The model under review builds one solid part; all positions refer to its coordinate system, in mm. A direction names the side the tool comes from. Coordinates: 2 decimals unless noted, no trailing zeros. Order: outer loops, then holes, each group sorted by start corner. A loop starts at its lowest first (then second) coordinate and runs counter-clockwise, first axis right, second up. Notation, with made-up numbers: M 26.25,9.5 L 84.25,9.5 A7 ccw 84.25,17.5 Z; hole C 77,30 d9. An arc over 180 degrees is marked long. Write each question's results on one line, items separated by ' | '.
from build123d import *

# Parameters (mm, degrees)
SKETCH1_W           = 120
SKETCH1_H           = 245
BOSS_EXTRUDE1_DEPTH = 42
CHAMFER1_SIZE       = 30
FILLET3_R           = 25
FILLET1_R           = 5
SHELL1_T            = -2


with BuildPart() as part:
    # Sketch1 → Boss-Extrude1 (new body)
    with BuildSketch(Plane.XY):
        with Locations((0, 72.5)):
            Rectangle(SKETCH1_W, SKETCH1_H)
    extrude(amount=BOSS_EXTRUDE1_DEPTH)

    # Chamfer1
    chamfer1_edges = [part.edges().sort_by_distance(p)[0] for p in [
        (60, -50, 21),
        (-60, -50, 21),
    ]]
    chamfer(chamfer1_edges, length=CHAMFER1_SIZE)

    # Fillet3
    fillet3_edges = [part.edges().sort_by_distance(p)[0] for p in [
        (30, -50, 21),
        (-30, -50, 21),
        (-60, -20, 21),
        (60, -20, 21),
    ]]
    fillet(fillet3_edges, radius=FILLET3_R)

    # Fillet1
    fillet1_edges = [part.edges().sort_by_distance(p)[0] for p in [
        (-45, -35, 0),
        (0, -50, 0),
        (60, 92.67766953, 0),
        (45, -35, 0),
        (58.096988313, -19.21174675, 0),
        (29.21174675, -48.096988313, 0),
        (-29.21174675, -48.096988313, 0),
        (-58.096988313, -19.21174675, 0),
        (0, 195, 0),
        (-60, 92.67766953, 0),
    ]]
    fillet(fillet1_edges, radius=FILLET1_R)

    # Shell1
    shell1_openings = [part.faces().sort_by_distance(p)[0] for p in [
        (0, 76.260599265, 42),
    ]]
    offset(amount=SHELL1_T, openings=shell1_openings)


solid = part.part
1) Take a section at B-B on x = 14. State the section outline as (y, z) points.
Solutions:
outline: M -50,5 A5 ccw -45,0 L 190,0 A5 ccw 195,5 L 195,42 L 193,42 L 193,5 A3 cw 190,2 L -45,2 A3 cw -48,5 L -48,42 L -50,42 Z
2) To check wall thickness, follow line 1 along Y through (x, z) = (-0.5, 6); line 2 along X through (y, z) = (132, 34); line 3 along Z through (x, y) = (18, -1.5). State the ranges of each line that lie inside material, in increasing order.
Solutions:
line 1: -50 to -48, 193 to 195 | line 2: -60 to -58, 58 to 60 | line 3: 0 to 2
3) Take a section at C-C on y = 23. State the section outline as (x, z) points, plus the area to 3 significant figures.
Solutions:
outline: M -60,5 A5 ccw -55,0 L 55,0 A5 ccw 60,5 L 60,42 L 58,42 L 58,5 A3 cw 55,2 L -55,2 A3 cw -58,5 L -58,42 L -60,42 Z | area: 393 mm2
4) For faces 5 (the cylindrical face through (58, 94, 1)), 6 (the flat face through (58, 90, 23)), list the 3-axis set-ups (+Z, -Z, +X, -X, +Y, -Y) from which the entire face can be reached by the end or side of a thin tool; tool diameter is ignored.
Solutions:
face 5: -Z, +X, +Y, -Y | face 6: +Z
5) For pin 1 (4 mm diameter, centred on x = 33.5, z = 22.5, fed in from -Y); pin 2 (5 mm diameter, centred on x = -17, y = 15, fed in from +Z), all flat-tipped, find the tip position at first contact; note any pin that passes through.
Solutions:
pin 1: y = -47.01 | pin 2: z = 2
6) Take a section at A-A on z = 26. State the section outline as (x, y) points.
Solutions:
outline: M -60,-9.64 A25 ccw -52.68,-27.32 L -37.32,-42.68 A25 ccw -19.64,-50 L 19.64,-50 A25 ccw 37.32,-42.68 L 52.68,-27.32 A25 ccw 60,-9.64 L 60,195 L -60,195 Z; hole M -58,-9.64 A23 ccw -51.26,-25.91 L -35.91,-41.26 A23 ccw -19.64,-48 L 19.64,-48 A23 ccw 35.91,-41.26 L 51.26,-25.91 A23 ccw 58,-9.64 L 58,193 L -58,193 Z
7) The part is to be moulded in two halves that separate along Y. For faces 1 (the flat face through (-1, 74, 0)), 2 (the cylindrical face through (1, 193, 1)), 3 (the cylindrical face through (-28.56, -46.2, 23.76)), 4 (the flat face through (-58, 90, 23)), say which applies: pulls with the +Y half, pulls with the -Y half, needs draft (parallel to the pull), parting line crosses it, or undercut.
Solutions:
face 1: needs draft | face 2: pulls with the +Y half | face 3: undercut | face 4: undercut
